from build123d import *

# Parameters (mm, degrees)
SKETCH1_W           = 80
SKETCH1_H           = 60
SKETCH1_R           = 16
BOSS_EXTRUDE1_DEPTH = 6
SCALE1_SCALE        = 7.5
SKETCH2_W           = 741.9419144
SKETCH2_H           = 114.286704827
CUT_EXTRUDE1_DEPTH  = 46


with BuildPart() as part:
    # Sketch1 → Boss-Extrude1 (new body)
    with BuildSketch(Plane(origin=(0, 0, 0), x_dir=(1, 0, 0), z_dir=(0, 1, 0))):
        with Locations((40, 30)):
            Rectangle(SKETCH1_W, SKETCH1_H)
        with Locations((49, 23.2)):
            Circle(SKETCH1_R, mode=Mode.SUBTRACT)
    extrude(amount=BOSS_EXTRUDE1_DEPTH)


with BuildPart() as part_1:
    # Scale1: scaled about (38.188518966, 3, -31.368674559)
    add(part.part.scale(SCALE1_SCALE).moved(Location((-248.225373279, -19.5, 203.896384633))))

    # Sketch2 → Cut-Extrude1 (cut, through all)
    with BuildSketch(Plane(origin=(0, 25.5, 0), x_dir=(1, 0, 0), z_dir=(0, 1, 0))):
        with Locations((57.597106318, 203.246967778)):
            Rectangle(SKETCH2_W, SKETCH2_H)
    extrude(amount=-CUT_EXTRUDE1_DEPTH, mode=Mode.SUBTRACT)


solid = part_1.part
The listing builds one solid part. Answer for the finished solid, in the listing's coordinates (mm). Give positions to 0.01 mm unless a question says otherwise; leave off trailing zeros. Write each loop counter-clockwise with the first axis right and the second up, starting at its lowest first coordinate (ties: lowest second). Pieces come first, ordered by that corner, then holes.
1) Section B-B (x = 33.5) is taken. Write down the section's boundary in (y, z).
2) For a pull along X with two mould halves and no side action, classify faces 1 (the face through (351.775, 3, 31)), 2 (the face through (24.047, 2.685, 102.915)), 3 (the face through (48, 3, -146.104)) as pulls with the +X half, pulls with the -X half, needs draft (parallel to the pull), parting line crosses it, or undercut.
3) Section A-A (z = 125) is taken. Write down the section's boundary in (x, y).
4) Section C-C (y = 10) is taken. Write down the section's boundary in (x, z), and give its area (3 significant figures).
5) Find the intervals of material crossed by L1, parallel to X at y = 17, z = 29.5; L2, parallel to X at y = 17.5, z = 32; L3, parallel to Z at x = 205, y = 9, in increasing order.
Response:
1. outline: (-19.5, -146.1) - (25.5, -146.1) - (25.5, -54.02) - (-19.5, -54.02) - close; (-19.5, 113.82) - (25.5, 113.82) - (25.5, 203.9) - (-19.5, 203.9) - close
2. face 1: pulls with the +X half
2. face 2: undercut
2. face 3: needs draft
3. outline: (-248.23, -19.5) - (46.09, -19.5) - (46.09, 25.5) - (-248.23, 25.5) - close; (192.45, -19.5) - (351.77, -19.5) - (351.77, 25.5) - (192.45, 25.5) - close
4. outline: (-248.23, -146.1) - (351.77, -146.1) - (351.77, 203.9) - (-248.23, 203.9) - close; hole circle Ø240 at (119.27, 29.9)
4. area: 165,000 mm2
5. L1: x = -248.23 to -0.72, 239.27 to 351.77
5. L2: x = -248.23 to -0.71, 239.26 to 351.77
5. L3: z = -146.1 to -54.07, 113.87 to 203.9
